Can you work these out from the model? Positions are in its coordinate system, mm. Round coordinates to 2 decimals unless told otherwise and drop trailing zeros. Loops run counter-clockwise (first coordinate to the right, second up) from the corner with the lowest first, then second, coordinate; pieces in that order, holes last. Notation, with made-up numbers: (84.25, 73.5) -> (120.25, 73.5) arc R28 ccw to (120.25, 111.5) -> close; hole circle Ø1 at (78, 81). An arc over 180 degrees is marked (long way). Write item = value, one per line.
from build123d import *

# Parameters (mm, degrees)
BOSS_EXTRUDE1_DEPTH  = 3
SKETCH11_OUTSIDE_W   = 186.736
SKETCH11_OUTSIDE_H   = 177.534
SKETCH11_OUTSIDE_W_2 = 80
SKETCH11_OUTSIDE_H_2 = 40
CUT_EXTRUDE13_DEPTH  = 103.574363269
SKETCH12_R           = 2.4
CUT_EXTRUDE15_DEPTH  = 83.856804186
SKETCH13_R           = 2.5
CUT_EXTRUDE16_DEPTH  = 83.856804186


with BuildPart() as part:
    # Sketch1 → Boss-Extrude1 (new body)
    with BuildSketch(Plane(origin=(0, 0, 0), x_dir=(1, 0, 0), z_dir=(0, 1, 0))):
        with BuildLine():
            ThreePointArc((36.543377003, -62.616544118), (0, 72.5), (-36.543377003, -62.616544118))
            ThreePointArc((-36.543377003, -62.616544118), (-33.085954668, -63.20954405), (-30.089832649, -61.38507948))
            ThreePointArc((-30.089832649, -61.38507948), (0, -46.75), (30.089832649, -61.38507948))
            ThreePointArc((30.089832649, -61.38507948), (33.085954668, -63.20954405), (36.543377003, -62.616544118))
        make_face()
    extrude(amount=BOSS_EXTRUDE1_DEPTH)

    # Sketch11 outside → Cut-Extrude13 (cut, through all)
    with BuildSketch(Plane.XZ):
        with Locations((0, -4.601)):
            Rectangle(SKETCH11_OUTSIDE_W, SKETCH11_OUTSIDE_H)
        with Locations((0, -57)):
            Rectangle(SKETCH11_OUTSIDE_W_2, SKETCH11_OUTSIDE_H_2, mode=Mode.SUBTRACT)
    extrude(amount=-CUT_EXTRUDE13_DEPTH, mode=Mode.SUBTRACT)

    # Sketch12 → Cut-Extrude15 (cut, through all)
    with BuildSketch(Plane.XZ):
        with Locations(Location((0, -65, 0), (0, 0, 270))):
            Circle(SKETCH12_R)
        with Locations(Location((0, -43, 0), (0, 0, 270))):
            Circle(SKETCH12_R)
    extrude(amount=-CUT_EXTRUDE15_DEPTH, mode=Mode.SUBTRACT)

    # Sketch13 → Cut-Extrude16 (cut, through all)
    with BuildSketch(Plane.XZ):
        with Locations(Location((0, -54, 0), (0, 0, 270))):
            Circle(SKETCH13_R)
    extrude(amount=-CUT_EXTRUDE16_DEPTH, mode=Mode.SUBTRACT)


solid = part.part
1. We'd pull the mould along X, two halves only. Please class faces 1 (the cylindrical face through (0.593, 1.479, -72.498)), 2 (the cylindrical face through (0.106, 1.479, -40.602)), 3 (the flat face through (40, 1, -49)), 4 (the cylindrical face through (-0.919, 1.479, -67.217)): released by +X, released by -X, zero draft, split by the parting line, or undercut.
Entries:
face_1 = split by the parting line
face_2 = undercut
face_3 = released by +X
face_4 = undercut
2. Suppose I cut it at A-A, the plane z = -43. List the corners of the cut face in (x, y) for me, and give its area (3 significant figures).
Entries:
outline = (-40, 0) -> (-2.4, 0) -> (-2.4, 3) -> (-40, 3) -> close; (2.4, 0) -> (40, 0) -> (40, 3) -> (2.4, 3) -> close
area = 226 mm²
3. Suppose I cut it at B-B, the plane x = 0. List the corners of the cut face in (y, z) for me.
Entries:
outline = (0, -72.5) -> (3, -72.5) -> (3, -67.4) -> (0, -67.4) -> close; (0, -62.6) -> (3, -62.6) -> (3, -56.5) -> (0, -56.5) -> close; (0, -51.5) -> (3, -51.5) -> (3, -45.4) -> (0, -45.4) -> close; (0, -40.6) -> (3, -40.6) -> (3, -37) -> (0, -37) -> close
4. Suppose I cut it at D-D, the plane z = -54. List the corners of the cut face in (x, y) for me.
Entries:
outline = (-40, 0) -> (-2.5, 0) -> (-2.5, 3) -> (-40, 3) -> close; (2.5, 0) -> (40, 0) -> (40, 3) -> (2.5, 3) -> close
5. I'm going to push a flat-ended pin straight in: pin 1 (1.5 mm diameter, centred on x = 26, y = 2, fed in from -Z). Where does the tip first touch, or does it pass through?
Entries:
pin_1 = -67.96
6. I need wall thicknesses on line 1 (X direction, y = 1.3, z = -54); line 2 (X direction, y = 1.45, z = -63.5); line 3 (X direction, y = 2.1, z = -67.5). Which ranges of each line are inside material? Lowest first, please. Write a range as [from, to].
Entries:
line_1 = [-40, -2.5], [2.5, 40]
line_2 = [-34.99, -1.87], [1.87, 34.99]
line_3 = [-26.46, 26.46]
7. Suppose I cut it at C-C, the plane y = 2.5. List the corners of the cut face in (x, z) for me, and give its area (3 significant figures).
Entries:
outline = (-40, -60.47) arc R72.5 ccw to (40, -60.47) -> (40, -37) -> (-40, -37) -> close; hole circle Ø5 at (0, -54); hole circle Ø4.8 at (0, -65); hole circle Ø4.8 at (0, -43)
area = 2,470 mm²
